Build history of the part. All positions in model axes, mm. Face numbers are marked on the shaded views. Coordinates: 2 decimals unless noted, no trailing zeros. Loops run counter-clockwise (first coordinate to the right, second up) from the corner with the lowest first, then second, coordinate; pieces in that order, holes last.
(1) Two-plate mould, pull along Z, no slides. Class the marked faces 1, 2 and 3: pulls with the +Z half, pulls with the -Z half, needs draft (parallel to the pull), parting line crosses it, or undercut.
(2) Slice it at D-D (x = -58). Give the cut face in (y, z), and give its area (3 significant figures).
(3) Wall check: L1, parallel to X at y = 1.2, z = -6; L2, parallel to Y at x = -71, z = -156.5. Give the ranges that are in metal, low to high.
(4) Slice it at C-C (z = -59). Give the cut face in (x, y), and give its area (3 significant figures).
(5) Slice it at B-B (x = -101). Give the cut face in (y, z).
(6) Flat gauge pins, fed straight in: P1, Ø1, axis at x = -135.5, y = 18.5, coming from the -Z side; P2, Ø6, axis at x = -144, y = 26, coming from the +Z side; P3, Ø12, axis at x = -136, y = 20.5, coming from the -Z side. Where does each tip first touch, or does it go through?
(7) Slice it at A-A (y = 14.25). Give the cut face in (x, z) (3 decimals).
Autodesk Inventor part; units mm, degrees
ref_plane "YZ Plane" through (0, 0, 0) normal (1, 0, 0) x (0, 1, 0)
ref_plane "XZ Plane" through (0, 0, 0) normal (0, 1, 0) x (-1, 0, 0)
ref_plane "XY Plane" through (0, 0, 0) normal (0, 0, 1) x (1, 0, 0)
sketch "Sketch1" plane through (0, 0, 0) normal (0, 1, 0) x (-1, 0, 0)
  line L0 (0, 0) -> (180, 0)
  line L1 (180, 0) -> (180, -180)
  line L2 (180, -180) -> (0, -180)
  line L3 (0, -180) -> (0, 0)
  dimension "d0" = 180
  dimension "d1" = 180
extrude "Extrusion1" add sketch "Sketch1" along normal blind 2
sketch "Sketch3" plane through (0, 2, 0) normal (0, 1, 0) x (1, 0, 0)
  circle A0 centre (-174, 6) radius 1.65
  circle A1 centre (-174, 174) radius 1.65
  circle A2 centre (-6, 174) radius 1.65
  circle A3 centre (-6, 6) radius 1.65
  point P0 (0, 0)
  dimension "d9" = 3.3
  dimension "d10" = 3.3
  dimension "d11" = 3.3
  dimension "d12" = 3.3
extrude "Extrusion3" cut sketch "Sketch3" against normal through all
sketch "Sketch10" plane through (0, 2, 0) normal (0, 1, 0) x (1, 0, 0)
  line L0 (0, 180) -> (-180, 180)
  circle A0 centre (-110.675, 90) radius 35.2
  circle A1 centre (-110.675, 90) radius 37.2
  circle A2 centre (-110.675, 90) radius 28 construction
  line L1 (-110.675, 90) -> (-73.475, 90) construction
  line L2 (-110.675, 90) -> (-129.275, 122.216145) construction
  line L3 (-90.675, 90) -> (-53.475, 90) construction
  line L4 (-110.675, 90) -> (-129.275, 57.783855) construction
  line L5 (-90.675, 90) -> (-53.475, 90) construction
  circle A3 centre (-124.675, 114.248711) radius 2.3
  circle A4 centre (-124.675, 114.248711) radius 4.3
  circle A5 centre (-124.675, 65.751289) radius 2.3
  circle A6 centre (-124.675, 65.751289) radius 4.3
  circle A7 centre (-82.675, 90) radius 2.3
  circle A8 centre (-82.675, 90) radius 4.3
  circle A9 centre (-110.675, 90) radius 33.2
  circle A10 centre (-110.675, 90) radius 23.7
  point P0 (0, 0)
  dimension "d68" = 70.4
  dimension "d69" = 74.4
  dimension "d70" = 56
  dimension "d71" = 120
  dimension "d72" = 120
  dimension "d73" = 4.6
  dimension "d74" = 8.6
  dimension "d75" = 4.6
  dimension "d76" = 8.6
  dimension "d77" = 4.6
  dimension "d78" = 8.6
  dimension "d79" = 66.4
  dimension "d88" = 47.4
sketch "Sketch10 outline for Extrusion11" plane through (0, 2, 0) normal (0, 1, 0) x (1, 0, 0)
  circle A0 centre (-110.675, 90) radius 35.2
  circle A1 centre (-110.675, 90) radius 33.2
  circle A2 centre (-82.675, 90) radius 4.3
  circle A3 centre (-82.675, 90) radius 2.3
  circle A4 centre (-124.675, 65.751289) radius 4.3
  circle A5 centre (-124.675, 65.751289) radius 2.3
  circle A6 centre (-124.675, 114.248711) radius 4.3
  circle A7 centre (-124.675, 114.248711) radius 2.3
extrude "Extrusion11" add sketch "Sketch10 outline for Extrusion11" along normal blind 20
sketch "Sketch10 outline for Extrusion12" plane through (0, 2, 0) normal (0, 1, 0) x (1, 0, 0)
  circle A0 centre (-110.675, 90) radius 37.2
  circle A1 centre (-110.675, 90) radius 35.2
extrude "Extrusion12" add sketch "Sketch10 outline for Extrusion12" along normal blind 28
sketch "Sketch10 outline for Extrusion13" plane through (0, 2, 0) normal (0, 1, 0) x (1, 0, 0)
  circle A0 centre (-110.675, 90) radius 23.7
extrude "Extrusion13" cut sketch "Sketch10 outline for Extrusion13" against normal through all
sketch "Sketch10 outline for Extrusion14" plane through (0, 2, 0) normal (0, 1, 0) x (1, 0, 0)
  circle A0 centre (-124.675, 114.248711) radius 2.3
  circle A1 centre (-124.675, 65.751289) radius 2.3
  circle A2 centre (-82.675, 90) radius 2.3
extrude "Extrusion14" cut sketch "Sketch10 outline for Extrusion14" against normal through all
properties part number "top plate"
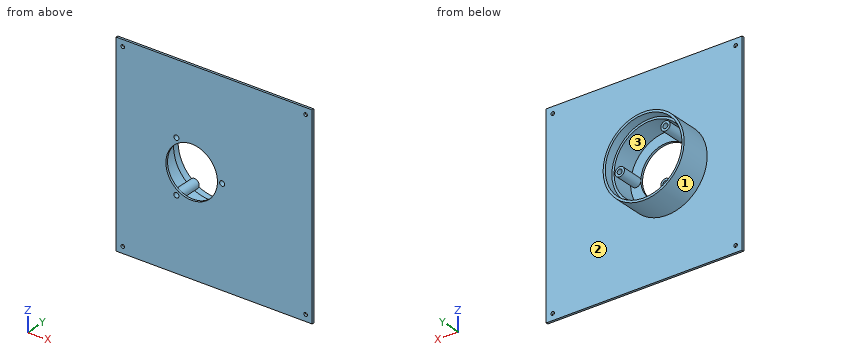
Response values:
1. face 1: parting line crosses it
1. face 2: needs draft
1. face 3: undercut
2. outline: (0, -180) - (2, -180) - (2, 0) - (0, 0) - close
2. area: 360 mm2
3. L1: x = -180 to -175.65, -172.35 to -7.65, -4.35 to 0
3. L2: y = 0 to 2
4. outline: (-180, 0) - (0, 0) - (0, 2) - (-90.11, 2) - (-90.11, 30) - (-94, 30) - (-94, 22) - (-98.79, 22) - (-98.79, 2) - (-122.56, 2) - (-122.56, 22) - (-127.35, 22) - (-127.35, 30) - (-131.24, 30) - (-131.24, 2) - (-180, 2) - close
4. area: 769 mm2
5. outline: (0, -180) - (2, -180) - (2, -125.92) - (30, -125.92) - (30, -123.84) - (22, -123.84) - (22, -121.76) - (2, -121.76) - (2, -111.64) - (0, -111.64) - close; (0, -68.36) - (2, -68.36) - (2, -58.24) - (22, -58.24) - (22, -56.16) - (30, -56.16) - (30, -54.08) - (2, -54.08) - (2, 0) - (0, 0) - close
6. P1: stops at z = -118.14
6. P2: stops at z = -68.45
6. P3: stops at z = -121.79
7. outline: circle Ø74.4 at (-110.675, -90); circle Ø8.6 at (-124.675, -114.249); circle Ø8.6 at (-124.675, -65.751); circle Ø8.6 at (-82.675, -90); hole circle Ø66.4 at (-110.675, -90); hole circle Ø4.6 at (-124.675, -114.249); hole circle Ø4.6 at (-124.675, -65.751); hole circle Ø4.6 at (-82.675, -90)
